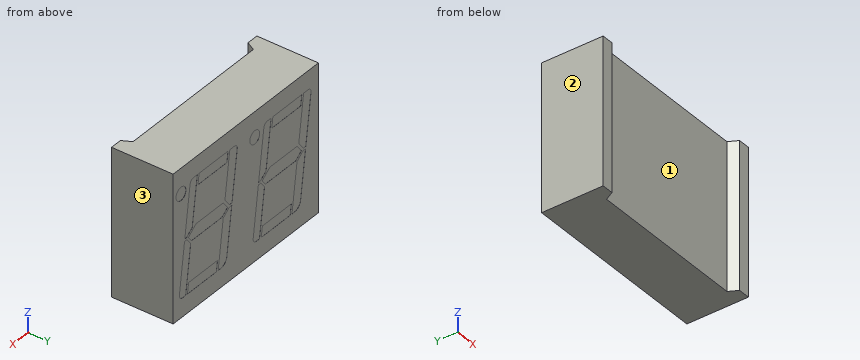
```python
from build123d import *

# Parameters (mm, degrees)
SKETCH1_W           = 25
SKETCH1_H           = 19.05
BOSS_EXTRUDE1_DEPTH = 8
CUT_EXTRUDE1_DEPTH  = 25.148550681
SKETCH3_R           = 0.85
CUT_EXTRUDE3_DEPTH  = 0.01
LPATTERN2_COUNT     = 2
LPATTERN2_PITCH     = 12.7


with BuildPart() as part:
    # Sketch1 → Boss-Extrude1 (new body)
    with BuildSketch(Plane(origin=(0, 0, 0), x_dir=(1, 0, 0), z_dir=(0, 1, 0))):
        Rectangle(SKETCH1_W, SKETCH1_H)
    extrude(amount=BOSS_EXTRUDE1_DEPTH)

    # Sketch2 → Cut-Extrude1 (cut, through all)
    with BuildSketch(Plane.XY.offset(9.525)):
        Polygon((-10.357683229, 1.165391541), (-10.979622637, 0), (10.979622637, 0), (10.357683229, 1.165391541), align=None)
    extrude(amount=-CUT_EXTRUDE1_DEPTH, mode=Mode.SUBTRACT)

    # Sketch3 → Cut-Extrude3 (cut)
    with BuildSketch(Plane(origin=(0, 8, 0), x_dir=(1, 0, 0), z_dir=(0, 1, 0))):
        with Locations(Location((-1.55, -6.26, 0), (0, 0, 270))):
            Circle(SKETCH3_R)
        with BuildLine():
            Line((-10.293918875, 0.15), (-9.446582946, 6.179108414))
            ThreePointArc((-9.446582946, 6.179108414), (-9.085171861, 6.844744827), (-8.375714675, 7.11))
            Line((-8.375714675, 7.11), (-7.952487442, 7.11))
            Line((-7.952487442, 7.11), (-8.820313991, 0.935093249))
            Line((-8.820313991, 0.935093249), (-9.862167922, 0.15))
            Line((-9.862167922, 0.15), (-10.293918875, 0.15))
        make_face()
        with BuildLine():
            Line((-2.367186588, 7.11), (-1.813478843, 7.11))
            ThreePointArc((-1.813478843, 7.11), (-1.401654728, 6.922320938), (-1.273116986, 6.488384791))
            Line((-1.273116986, 6.488384791), (-2.163918875, 0.15))
            Line((-2.163918875, 0.15), (-2.593918875, 0.15))
            Line((-2.593918875, 0.15), (-3.227234844, 0.990438678))
            Line((-3.227234844, 0.990438678), (-2.367186588, 7.11))
        make_face()
        Polygon((-7.652487442, 7.11), (-2.667186588, 7.11), (-2.856916715, 5.76), (-7.842217569, 5.76), align=None)
        Polygon((-8.604632176, 0.726571417), (-3.369972607, 0.726571417), (-2.822461773, 0), (-4.142522346, -0.994736992), (-8.819236923, -0.994736992), (-9.568825012, 0), align=None)
        with BuildLine():
            Line((-10.336081125, -0.15), (-9.904330172, -0.15))
            Line((-9.904330172, -0.15), (-9.119236923, -1.191853931))
            Line((-9.119236923, -1.191853931), (-9.950978112, -7.11))
            Line((-9.950978112, -7.11), (-10.750461652, -7.11))
            ThreePointArc((-10.750461652, -7.11), (-11.120337027, -6.94143808), (-11.235781811, -6.551703021))
            Line((-11.235781811, -6.551703021), (-10.336081125, -0.15))
        make_face()
        Polygon((-9.650978112, -7.11), (-4.665677257, -7.11), (-4.47594713, -5.76), (-9.461247985, -5.76), align=None)
        with BuildLine():
            Line((-2.206081125, -0.15), (-3.108270084, -6.569408002))
            ThreePointArc((-3.108270084, -6.569408002), (-3.318150529, -6.955959695), (-3.730150039, -7.11))
            Line((-3.730150039, -7.11), (-4.365677257, -7.11))
            Line((-4.365677257, -7.11), (-3.489911075, -0.878599823))
            Line((-3.489911075, -0.878599823), (-2.523026453, -0.15))
            Line((-2.523026453, -0.15), (-2.206081125, -0.15))
        make_face()
    cut_extrude3 = extrude(amount=-CUT_EXTRUDE3_DEPTH, mode=Mode.SUBTRACT)

    # LPattern2: Cut-Extrude3 ×2
    with Locations(*[(i * LPATTERN2_PITCH, 0, 0) for i in range(1, LPATTERN2_COUNT)]):
        add(cut_extrude3, mode=Mode.SUBTRACT)


solid = part.part
```
The model under review builds one solid part; all positions refer to its coordinate system, in mm. Face numbers are marked on the shaded views. Give positions to 0.01 mm unless a question says otherwise; leave off trailing zeros. Write each loop counter-clockwise with the first axis right and the second up, starting at its lowest first coordinate (ties: lowest second). Pieces come first, ordered by that corner, then holes. Notation, with made-up numbers: (57, 20.5) - (98, 20.5) arc R13 ccw to (98, 37.5) - close; hole circle Ø7 at (43.5, 32.25). An arc over 180 degrees is marked (long way). Answer in a Markdown table with one row per item. Add a question column.
1. Draft analysis for pull direction X (two halves, no side actions). For the marked faces 1, 2 and 3, state which applies: +X half, -X half, draft (parallel to the pull), parting line (faces both ways), or undercut.
2. We need section A-A on z = -8. Write out the cut boundary in (x, y).
3. Insertion check: P1, Ø1.9, axis at x = -7, z = 0, coming from the +Y side. The pin has a flat end and moves straight along its axis. Give the tip position at first contact, or say it passes through.
4. We need section B-B on x = 0.25. Write out the cut boundary in (y, z) (3 decimals).
5. Wall thickness on line 1 along Y through (x, z) = (10, -1.75); line 2 along Y through (x, z) = (11, -3.5); line 3 along X through (y, z) = (0.5, 8): over which ranges is each line inside the solid? List them lowest first. Write a range as [from, to].
Ans:
| question | item | result |
|---|---|---|
| 1 | face 1 | undercut |
| 1 | face 2 | -X half |
| 1 | face 3 | +X half |
| 2 | outline | (-12.5, 0) - (-10.98, 0) - (-10.36, 1.17) - (10.36, 1.17) - (10.98, 0) - (12.5, 0) - (12.5, 8) - (-12.5, 8) - close |
| 3 | P1 | stops at y = 8 |
| 4 | outline | (1.165, -9.525) - (8, -9.525) - (8, 9.525) - (1.165, 9.525) - close |
| 5 | line 1 | y = [1.17, 7.99] |
| 5 | line 2 | y = [0, 7.99] |
| 5 | line 3 | x = [-12.5, -10.71], [10.71, 12.5] |
